from build123d import *

# Parameters (mm, degrees)
F0_R     = 2.9
F0_R_2   = 1.5
F1_DEPTH = 22.11
F2_START = 7
F0_R_3   = 3.4
F2_DEPTH = 10.7
F3_START = 5.2
F3_DEPTH = 1.8
F5_D     = 2.1
F6_D     = 4.1
F6_DEPTH = 4.4
F6_TIP   = 1.231764269
F7_SIZE  = 0.2


with BuildPart() as f1:
    # F0 (on Top) → F1 (new body)
    with BuildSketch(Plane.XY):
        Circle(F0_R)
        Circle(F0_R_2, mode=Mode.SUBTRACT)
        Circle(F0_R_2)
    extrude(amount=F1_DEPTH)

    # F0 (on Top) → F2 (join)
    with BuildSketch(Plane.XY.offset(F2_START)):
        Circle(F0_R_3)
        Circle(F0_R, mode=Mode.SUBTRACT)
    extrude(amount=F2_DEPTH)

    # F0 (on Top) → F3 (cut)
    with BuildSketch(Plane.XY.offset(F3_START)):
        Circle(F0_R_3)
        Circle(F0_R, mode=Mode.SUBTRACT)
        Circle(F0_R)
        Circle(F0_R_2, mode=Mode.SUBTRACT)
    extrude(amount=F3_DEPTH, mode=Mode.SUBTRACT)

    # F5 (through all)
    with Locations(Plane.XY.offset(22.11)):
        with Locations((0, 0)):
            Hole(F5_D / 2)

    # F6
    with Locations(Plane.XY.offset(22.11)):
        with Locations((0, 0)):
            Hole(F6_D / 2, depth=F6_DEPTH)
            with Locations((0, 0, -(F6_DEPTH + F6_TIP / 2))):  # 118° drill point
                Cone(0, F6_D / 2, F6_TIP, mode=Mode.SUBTRACT)

    # F7
    f7_edges = [f1.edges().sort_by_distance(p)[0] for p in [
        (-2.9, 0, 22.11),
        (-2.9, 0, 5.2),
        (-2.9, 0, 0),
        (-3.4, 0, 7),
        (-3.4, 0, 17.7),
        (-2.05, 0, 22.11),
    ]]
    chamfer(f7_edges, length=F7_SIZE)


solid = f1.part
Check sheet for the modelled part. Datum: model origin and axes. Units: mm. A direction names the side the tool comes from. Give positions to 0.01 mm unless a question says otherwise; leave off trailing zeros. Loops run counter-clockwise (first coordinate to the right, second up) from the corner with the lowest first, then second, coordinate; pieces in that order, holes last. Notation, with made-up numbers: M 30,30.25 L 85,30.25 A19 ccw 85,64.25 Z; hole C 82,89 d5. An arc over 180 degrees is marked long. Use a Markdown table: item, result. Add a question column.
Q1. Tool access check on faces 4 (the flat face through (-1.5, -0.7, 7)), 5 (the cylindrical face through (-1, 0.32, 8.43)), 6 (the cylindrical face through (-2.9, 0.1, 19.8)). Record the directions out of +Z, -Z, +X, -X, +Y, -Y that give a thin tool (end or side, any length) a straight path to the whole face; none if there is none.
Q2. Mould release check, pull along X, two halves, no side actions. Record for faces 1 (the cylindrical face through (-2.9, 0.1, 2.6)), 2 (the flat face through (1, -1, 0)), 3 (the cylindrical face through (0.267, 2.033, 19.781)): pulls with the +X half, pulls with the -X half, needs draft (parallel to the pull), parting line crosses it, or undercut.
Q3. Sectioned sample at A-A, the plane z = 15. Record the cut outline in (x, y), then the cut area to 3 significant figures.
Q4. Scan lines: line 1 along Y through (x, z) = (0, 18.8); line 2 along Z through (x, y) = (0.75, 2.5); line 3 along Y through (x, z) = (0, 11.5). Record each from-to range of solid material in increasing order. Write a range as [from, to].
Q5. Go/stop test with flat-tipped pins: pin 1 (1.7 mm diameter, centred on x = 0, y = 0, fed in from -Z); pin 2 (3 mm diameter, centred on x = -0.5, y = 1.5, fed in from +Z); pin 3 (1.5 mm diameter, centred on x = 1.5, z = 13.5, fed in from +Y); pin 4 (2 mm diameter, centred on y = 2, z = 18, fed in from +X). Record where each tip stops, or that it passes through.
Verdict:
| question | item | result |
|---|---|---|
| 1 | face 4 | none |
| 1 | face 5 | +Z, -Z |
| 1 | face 6 | +Z |
| 2 | face 1 | parting line crosses it |
| 2 | face 2 | needs draft |
| 2 | face 3 | undercut |
| 3 | outline | C 0,0 d6.8; hole C 0,0 d2.1 |
| 3 | area | 32.9 mm^2 |
| 4 | line 1 | [-2.9, -2.05], [2.05, 2.9] |
| 4 | line 2 | [0, 5.2], [7, 22.11] |
| 4 | line 3 | [-3.4, -1.05], [1.05, 3.4] |
| 5 | pin 1 | through |
| 5 | pin 2 | z = 22.11 |
| 5 | pin 3 | y = 3.32 |
| 5 | pin 4 | x = 3.21 |
